```python
from build123d import *

# Parameters (mm, degrees)
BOSS_EXTRUDE1_DEPTH = 6


with BuildPart() as part:
    # Sketch1 → Boss-Extrude1 (new body)
    with BuildSketch(Plane.XZ.offset(-7.628326304)):
        with BuildLine():
            Line((81.876098577, 72.144512579), (39.196222867, 54.502914987))
            ThreePointArc((39.196222867, 54.502914987), (34.956549827, 48.163081659), (39.196222867, 41.823248331))
            Line((39.196222867, 41.823248331), (81.876098577, 24.18165074))
            Line((81.876098577, 24.18165074), (81.923583987, 24.162022789))
            ThreePointArc((81.923583987, 24.162022789), (117.776549827, 48.163081659), (81.923583987, 72.164140529))
            Line((81.923583987, 72.164140529), (81.876098577, 72.144512579))
        make_face()
        with BuildLine():
            Line((82.186737097, 24.863925245), (39.481862188, 42.514347463))
            ThreePointArc((39.481862188, 42.514347463), (35.704351827, 48.163081659), (39.481862188, 53.811815856))
            Line((39.481862188, 53.811815856), (82.186737097, 71.462238074))
            ThreePointArc((82.186737097, 71.462238074), (117.027340827, 48.163081659), (82.186737097, 24.863925245))
        make_face(mode=Mode.SUBTRACT)
    extrude(amount=BOSS_EXTRUDE1_DEPTH)


solid = part.part
```
Geometry: final body of the model. Coordinates: model frame, mm. A direction names the side the tool comes from. Give positions to 0.01 mm unless a question says otherwise; leave off trailing zeros. Order: outer loops, then holes, each group sorted by start corner. A loop starts at its lowest first (then second) coordinate and runs counter-clockwise, first axis right, second up. Notation, with made-up numbers: M 36.5,35.25 L 48.5,35.25 A24 cw 48.5,57.25 Z; hole C -40,-39 d9. An arc over 180 degrees is marked long. Answer as CSV lines item,"result". Start each with the question number.
1) Set-up query: faces 4 (the flat face through (61.133, 4.67, 33.566)), 5 (the cylindrical face through (34.957, 4.67, 48.276)). Return all of +Z, -Z, +X, -X, +Y, -Y with unobstructed straight access to the full face (end or side cutting, diameter ignored); none if empty.
2) Line query: line 1 (X direction, y = 2.3, z = 62); line 2 (Z direction, x = 80, y = 4.4); line 3 (X direction, y = 7, z = 61). Output: solid intervals per line, ascending. Write a range as from..to.
3) Cut plane C-C (y = 6.6). Output: boundary loops of the cut face in (x, z), then the cut area to 3 significant figures.
4) Cut plane B-B (x = 69). Output: boundary loops of the cut face in (y, z), then the cut area to 3 significant figures.
5) Mould query, pull axis Z, two halves, no side actions, for faces 1 (the cylindrical face through (35.705, 4.67, 48.062)), 2 (the flat face through (66.97, 1.628, 30.98)), 3 (the cylindrical face through (117.767, 4.67, 47.45)). Classes: +Z half, -Z half, draft (parallel to the pull), parting line (faces both ways), or undercut.
6) Cut plane A-A (z = 63). Output: boundary loops of the cut face in (x, y), then the cut area to 3 significant figures.
7) First-contact query: P1, Ø3, axis at y = 5.5, z = 42, coming from the +X side; P2, Ø3, axis at x = 95.5, y = 3.5, coming from the -Z side; P3, Ø1.5, axis at y = 2.5, z = 55.5, coming from the -X side. Flat tips, straight axial feed; report the tip coordinate or a pass-through.
Findings below:
1,face 4,"+Y, -Y"
1,face 5,"-X, +Y, -Y"
2,line 1,"x = 57.33..59.29, 112.89..113.78"
2,line 2,"z = 24.96..25.77, 70.56..71.37"
2,line 3,"x = 54.91..56.87, 113.51..114.38"
3,outline,"M 39.2,41.82 L 81.92,24.16 A25.96 ccw long 81.92,72.16 L 39.2,54.5 A6.86 ccw Z; hole M 39.48,42.51 L 82.19,24.86 A25.21 ccw long 82.19,71.46 L 39.48,53.81 A6.11 ccw Z"
3,area,"156 mm²"
4,outline,"M 1.63,29.5 L 7.63,29.5 L 7.63,30.31 L 1.63,30.31 Z; M 1.63,66.01 L 7.63,66.01 L 7.63,66.82 L 1.63,66.82 Z"
4,area,"9.72 mm²"
5,face 1,"undercut"
5,face 2,"draft"
5,face 3,"parting line"
6,outline,"M 59.75,1.63 L 61.71,1.63 L 61.71,7.63 L 59.75,7.63 Z; M 112.2,1.63 L 113.12,1.63 L 113.12,7.63 L 112.2,7.63 Z"
6,area,"17.3 mm²"
7,P1,"stops at x = 117.35"
7,P2,"stops at z = 22.3"
7,P3,"stops at x = 39.79"
